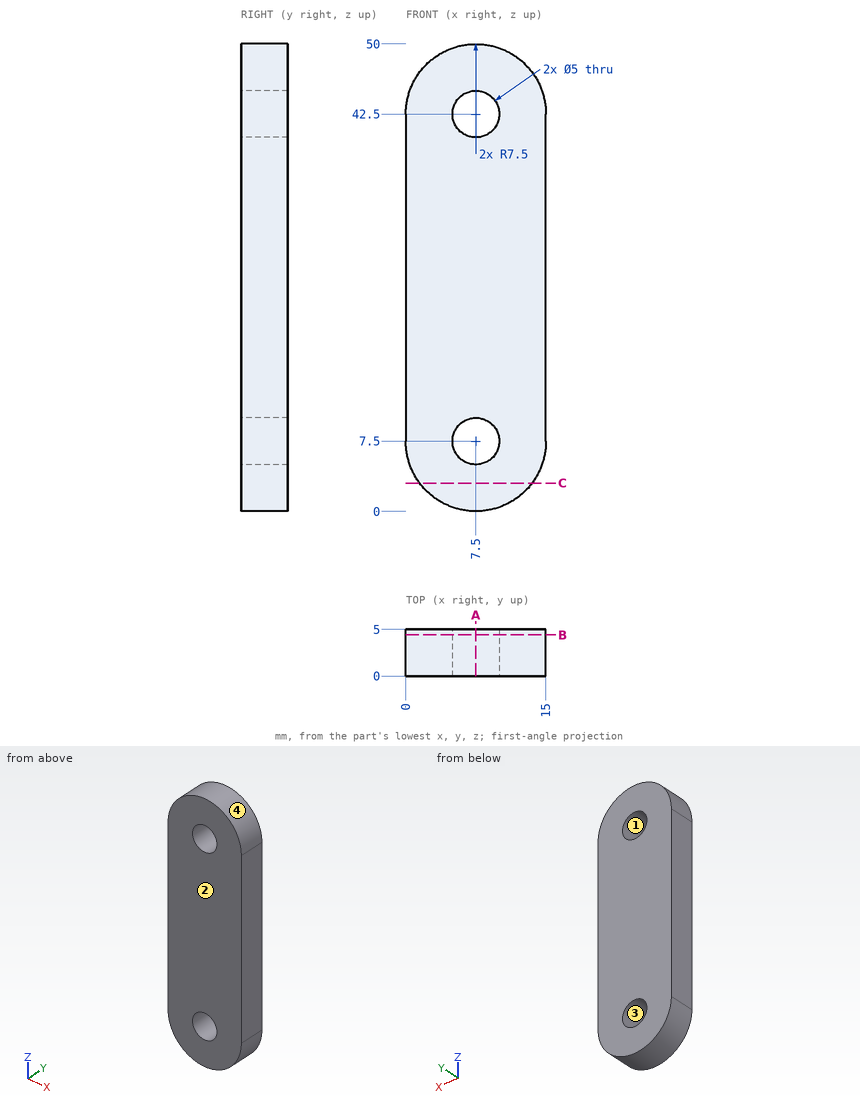
Geometry: see drawing. Coordinates: mm, zero at the bounding-box minimum. Coordinates: 2 decimals unless noted, no trailing zeros. Write each loop counter-clockwise with the first axis right and the second up, starting at its lowest first coordinate (ties: lowest second). Pieces come first, ordered by that corner, then holes.
1) Material intervals for line 1 along Z through (x, y) = (7.5, 2.25); line 2 along Z through (x, y) = (6.25, 3); line 3 along Z through (x, y) = (13.5, 3.8), sorted ascending.
2) Pin query (flat end, axial travel): pin 1 Ø3 at (x, z) = (7.5, 7.5) entering from -Y. Return the tip coordinate at first contact, or that it passes through.
3) Section A-A on x = 7.5. Output: boundary loops of the cut face in (y, z).
4) Section C-C on z = 3. Output: boundary loops of the cut face in (x, y), and give its area (3 significant figures).
5) Mould query, pull axis X, two halves, no side actions, for the marked faces 1, 2, 3 and 4. Classes: pulls with the +X half, pulls with the -X half, needs draft (parallel to the pull), parting line crosses it, or undercut.
6) Section B-B on y = 4.4. Output: boundary loops of the cut face in (x, z), and give its area (3 significant figures).
Check result:
1. line 1: z = 0 to 5, 10 to 40, 45 to 50
1. line 2: z = 0.1 to 5.33, 9.67 to 40.33, 44.67 to 49.9
1. line 3: z = 3 to 47
2. pin 1: passes through
3. outline: (0, 0) - (5, 0) - (5, 5) - (0, 5) - close; (0, 10) - (5, 10) - (5, 40) - (0, 40) - close; (0, 45) - (5, 45) - (5, 50) - (0, 50) - close
4. outline: (1.5, 0) - (13.5, 0) - (13.5, 5) - (1.5, 5) - close
4. area: 60.0 mm2
5. face 1: undercut
5. face 2: needs draft
5. face 3: undercut
5. face 4: parting line crosses it
6. outline: (0, 7.5) arc R7.5 ccw to (15, 7.5) - (15, 42.5) arc R7.5 ccw to (0, 42.5) - close; hole circle Ø5 at (7.5, 7.5); hole circle Ø5 at (7.5, 42.5)
6. area: 662 mm2
